The listing builds one solid part. Answer for the finished solid, in the listing's coordinates (mm). Face numbers are marked on the shaded views. A direction names the side the tool comes from. Round coordinates to 2 decimals unless told otherwise and drop trailing zeros. Loops run counter-clockwise (first coordinate to the right, second up) from the corner with the lowest first, then second, coordinate; pieces in that order, holes last. Notation, with made-up numbers: (69.5, 48) - (78.5, 48) arc R24 cw to (78.5, 65) - close; hole circle Ø10 at (80.25, -32). An arc over 180 degrees is marked (long way). Write item = value, one per line. Start each with the question number.
1) Section D-D, the plane z = 24.5 is taken. Determine the outline of the cut face in (x, y) (3 decimals).
2) A tool of negligible diameter and unlimited length cuts with its end or side. For the marked faces 1, 2 and 3, from which of +Z, -Z, +X, -X, +Y, -Y can it reach the whole face along a straight path? Write none if from no direction.
3) For a pull along X with two mould halves and no side action, classify the marked faces 4, 5 and 6 as released by +X, released by -X, zero draft, split by the parting line, or undercut.
4) Section B-B, the plane z = 28.5 is taken. Give the number of separate pieces and of enclosed holes in the cut face, and give its area (3 significant figures).
5) Given pin 1 Ø7 at (x, y) = (6, 11.5) entering from -Z; pin 2 Ø5 at (x, y) = (-15.5, 6) entering from +Z; pin 3 Ø4 at (x, y) = (4.74, 10.72) entering from -Z, each flat-ended and moving along its own axis, determine where each tip first touches the part or whether it passes through.
6) Section A-A, the plane z = 10.16 is taken. Determine the outline of the cut face in (x, y).
7) Section C-C, the plane y = -5 is taken. Determine the outline of the cut face in (x, z) (3 decimals).
8) Straight lines are drawn through the part: line 1 along X through (y, z) = (16, 14); line 2 along Y through (x, z) = (3, 11.5); line 3 along X through (y, z) = (9, 22.5). For each, find the intervals that lie inside material, in ascending order.
from build123d import *

# Parameters (mm, degrees)
F0_W      = 76.2
F0_H      = 38.1
F1_DEPTH  = 25.4
F2_SIZE   = 5.08
F3_R      = 11.1125
F4_DEPTH  = 12.7
F5_SIZE   = 3.175
F7_T      = 7.9375
F6_R      = 3.175
F8_DEPTH  = 7.9375
F9_R      = 3.175
F10_DEPTH = 7.9375


# Not quite as in the source:
# - a shell that OpenCascade refuses in one call is made with other operations: the cavity is built on its own and cut out


with BuildPart() as f1:
    # F0 (on Top) → F1 (new body)
    with BuildSketch(Plane.XY):
        with Locations((-12.72226125, 10.7161214997)):
            Rectangle(F0_W, F0_H)
    extrude(amount=F1_DEPTH)

    # F2
    f2_edges = [f1.edges().sort_by_distance(p)[0] for p in [
        (-50.822261, 10.716121, 25.4),
        (-12.722261, 29.766121, 25.4),
        (-12.722261, -8.333879, 25.4),
        (25.377739, 10.716121, 25.4),
    ]]
    chamfer(f2_edges, length=F2_SIZE)

    # F3 (on face) → F4 (join)
    with BuildSketch(Plane.XY.offset(25.4)):
        with Locations((-30.18476125, 10.7161214997)):
            Circle(F3_R)
        with Locations((4.74023875, 10.7161214997)):
            Circle(F3_R)
    extrude(amount=F4_DEPTH)

    # F5
    f5_edges = [f1.edges().sort_by_distance(p)[0] for p in [
        (-41.297261, 10.716121, 38.1),
        (-6.372261, 10.716121, 38.1),
    ]]
    chamfer(f5_edges, length=F5_SIZE)

    # F7: shell of thickness 7.9375, made by hand


with BuildPart() as f7_core1:
    # F7_t2: copy of F1
    add(f1.part)

    # the walls: a layer under each face that stays
    f7_faces = [f7_core1.faces().sort_by_distance(p)[0] for p in [
        (-41.29726125, 10.7161214997, 30.1625),
        (-39.70976125, 10.7161214997, 36.5125),
        (-12.72226125, 10.7161214997, 25.4),
        (-30.18476125, 10.7161214997, 38.1),
        (-48.28226125, 10.7161214997, 22.86),
        (-12.72226125, 27.2261214997, 22.86),
        (-12.72226125, -5.7938785003, 22.86),
        (22.83773875, 10.7161214997, 22.86),
        (-6.37226125, 10.7161214997, 30.1625),
        (-50.82226125, 10.7161214997, 10.16),
        (-12.72226125, 29.7661214997, 10.16),
        (-12.72226125, -8.3338785003, 10.16),
        (25.37773875, 10.7161214997, 10.16),
        (-4.78476125, 10.7161214997, 36.5125),
        (4.74023875, 10.7161214997, 38.1),
    ]]
    thicken(f7_faces, amount=-F7_T, mode=Mode.SUBTRACT)

    # F7_s3 → F7_t4 (revolve, cut)
    with BuildSketch(Plane.XZ.offset(-10.7161214997)):
        Polygon((-18.99288625, 25.479375), (-27.00976125, 25.4), (-27.00976125, 17.4625), (-19.07226125, 17.4625), align=None)
    revolve(axis=Axis((-30.18476125, 10.7161214997, 25.4), (0, 0, 1)), mode=Mode.SUBTRACT)

    # F7_s5 → F7_t6 (revolve, cut)
    with BuildSketch(Plane.XZ.offset(-10.7161214997)):
        Polygon((15.93211375, 25.479375), (15.85273875, 17.4625), (7.91523875, 17.4625), (7.91523875, 25.4), align=None)
    revolve(axis=Axis((4.74023875, 10.7161214997, 25.4), (0, 0, 1)), mode=Mode.SUBTRACT)


with BuildPart() as f1_1:
    add(f1.part)

    # what is left inside the walls is the cavity
    f7_cavity = [f7_core1.part.solids().sort_by_distance(p)[0] for p in [
        (-12.722261, 7.011955, 0.079375),
    ]]
    add(f7_cavity, mode=Mode.SUBTRACT)

    # F6 (on face) → F8 (cut)
    with BuildSketch(Plane.XZ.offset(8.3338785003)):
        with Locations((-12.72226125, 10.16)):
            Circle(F6_R)
    extrude(amount=-F8_DEPTH, mode=Mode.SUBTRACT)

    # F9 (on face) → F10 (cut)
    with BuildSketch(Plane(origin=(0, 29.7661214997, 0), x_dir=(-1, 0, 0), z_dir=(0, 1, 0))):
        with Locations((12.72226125, 10.16)):
            Circle(F9_R)
    extrude(amount=-F10_DEPTH, mode=Mode.SUBTRACT)


solid = f1_1.part
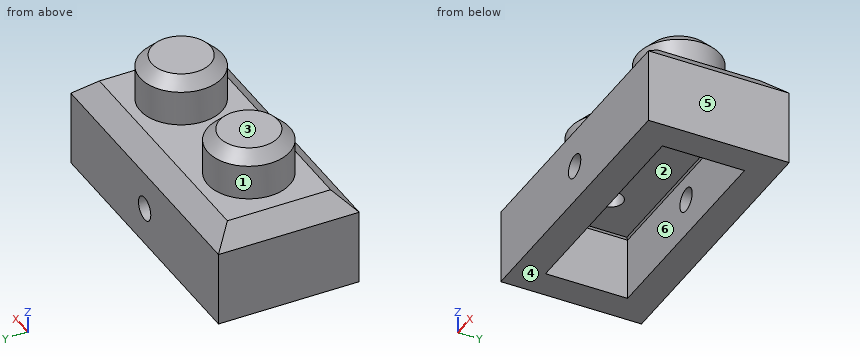
Geometry check:
q1.outline = (-46.642, -4.154) - (21.198, -4.154) - (21.198, 25.586) - (-46.642, 25.586) - close; hole circle Ø6.35 at (-30.185, 10.716); hole circle Ø6.35 at (4.74, 10.716)
q2.face_1 = +Z
q2.face_2 = -Z
q2.face_3 = +Z, +X, -X, +Y, -Y
q3.face_4 = zero draft
q3.face_5 = released by +X
q3.face_6 = undercut
q4.separate_pieces = 2
q4.enclosed_holes = 2
q4.area = 713 mm2
q5.pin_1 = 17.46
q5.pin_2 = 25.4
q5.pin_3 = 30.16
q6.outline = (-50.82, -8.33) - (-15.9, -8.33) - (-15.9, -0.4) - (-42.88, -0.4) - (-42.88, 21.83) - (-15.9, 21.83) - (-15.9, 29.77) - (-50.82, 29.77) - close; (-9.55, -8.33) - (25.38, -8.33) - (25.38, 29.77) - (-9.55, 29.77) - (-9.55, 21.83) - (17.44, 21.83) - (17.44, -0.4) - (-9.55, -0.4) - close
q7.outline = (-50.822, 0) - (25.378, 0) - (25.378, 20.32) - (22.044, 23.654) - (-47.488, 23.654) - (-50.822, 20.32) - close; hole circle Ø6.35 at (-12.722, 10.16)
q8.line_1 = -50.82 to -42.88, 17.44 to 25.38
q8.line_2 = -8.33 to -0.4, 21.83 to 29.77
q8.line_3 = -48.64 to -32.86, -27.51 to 2.07, 7.41 to 23.2
